Job drawing, mm, ordinate dimensions from the low corner. One solid piece. A direction names the side the tool comes from. Coordinates: 2 decimals unless noted, no trailing zeros. Write each loop counter-clockwise with the first axis right and the second up, starting at its lowest first coordinate (ties: lowest second). Pieces come first, ordered by that corner, then holes.
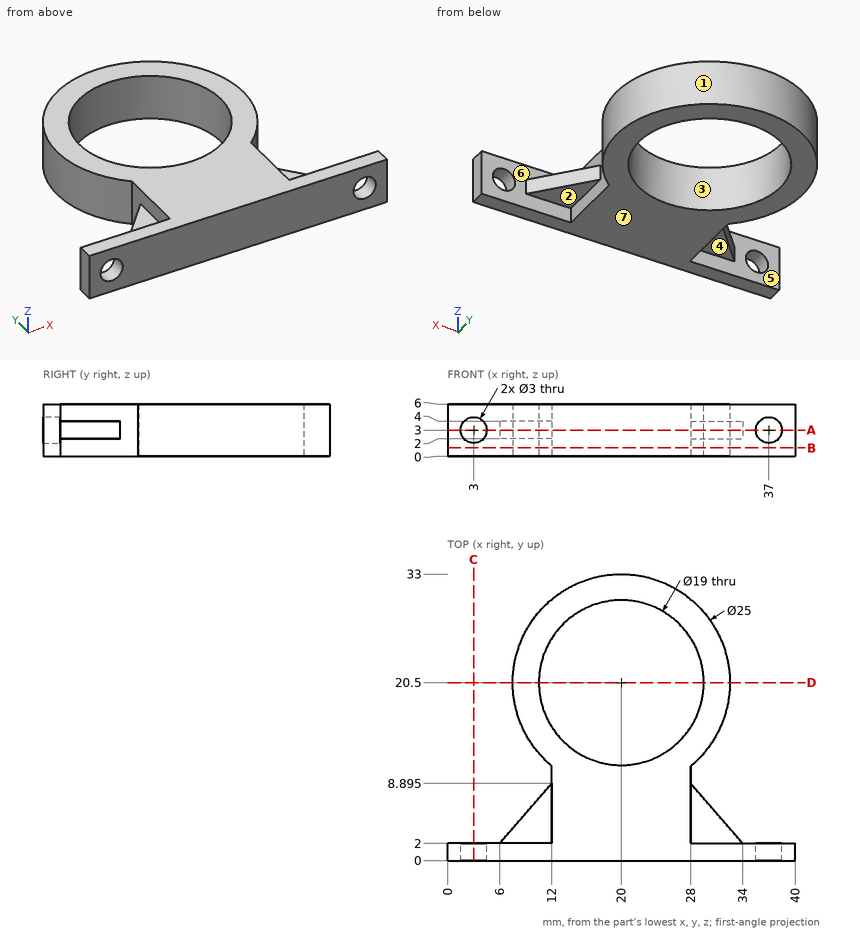
1. 3-axis set-ups, long thin cutter, end or side, ignore diameter. For the marked faces 4, 5, 6 and 7: which of +Z, -Z, +X, -X, +Y, -Y reach the whole face in a straight line?
Computed values:
face 4: -Z, -X
face 5: -X
face 6: +X
face 7: -Z, +X, -X, +Y, -Y
2. Saw through at A-A on z = 3. List the corners of the cut face in (x, y) (1 decimal), plus the area to 3 significant figures.
Computed values:
outline: (0, 0) - (1.5, 0) - (1.5, 2) - (0, 2) - close; (4.5, 0) - (35.5, 0) - (35.5, 2) - (34, 2) - (28, 8.9) - (28, 10.9) arc R12.5 ccw (long way) to (12, 10.9) - (12, 8.9) - (6, 2) - (4.5, 2) - close; (38.5, 0) - (40, 0) - (40, 2) - (38.5, 2) - close; hole circle Ø19 at (20, 20.5)
area: 427 mm2
3. Flat gauge pins, fed straight in: pin 1 (3 mm diameter, centred on x = 33, z = 1.5, fed in from +Y); pin 2 (3 mm diameter, centred on x = 30, y = 6.5, fed in from -Z); pin 3 (1.8 mm diameter, centred on y = 8, z = 3, fed in from -X); pin 4 (1.8 mm diameter, centred on x = 37, z = 3, fed in from +Y). Where does each tip first touch, or does it go through?
Computed values:
pin 1: stops at y = 25.4
pin 2: stops at z = 2
pin 3: stops at x = 10.44
pin 4: passes through
4. Saw through at D-D on y = 20.5. List the corners of the cut face in (x, z).
Computed values:
outline: (7.5, 0) - (10.5, 0) - (10.5, 6) - (7.5, 6) - close; (29.5, 0) - (32.5, 0) - (32.5, 6) - (29.5, 6) - close
5. Mould opens along X. For the marked faces 1, 2 and 3 say: +X half, -X half, draft (parallel to the pull), parting line (faces both ways), or undercut.
Computed values:
face 1: parting line
face 2: draft
face 3: undercut
6. Probe line 1 along X through (y, z) = (0.5, 3); line 2 along Y through (x, z) = (20, 3.35); line 3 along Y through (x, z) = (4, 5.2). List the from-to ranges inside material, lowest first.
Computed values:
line 1: x = 0 to 1.5, 4.5 to 35.5, 38.5 to 40
line 2: y = 0 to 11, 30 to 33
line 3: y = 0 to 2
7. Saw through at C-C on x = 3. List the corners of the cut face in (y, z).
Computed values:
outline: (0, 0) - (2, 0) - (2, 1.5) - (0, 1.5) - close; (0, 4.5) - (2, 4.5) - (2, 6) - (0, 6) - close
8. Saw through at B-B on z = 0.95. List the corners of the cut face in (x, y) (1 decimal), plus the area to 3 significant figures.
Computed values:
outline: (0, 0) - (40, 0) - (40, 2) - (28, 2) - (28, 10.9) arc R12.5 ccw (long way) to (12, 10.9) - (12, 2) - (0, 2) - close; hole circle Ø19 at (20, 20.5)
area: 398 mm2
